Part model, mm, in its own coordinate system. A direction names the side the tool comes from. Give positions to 0.01 mm unless a question says otherwise; leave off trailing zeros. Order: outer loops, then holes, each group sorted by start corner. A loop starts at its lowest first (then second) coordinate and runs counter-clockwise, first axis right, second up. Notation, with made-up numbers: (46.5, -4) - (93.5, -4) arc R20 cw to (93.5, 25) - close; hole circle Ø6 at (81.5, -17.75). An arc over 180 degrees is marked (long way). Use one line per item in the form item = value. Start each with the question number.
1. Pin check, flat tips, straight feed: P1, Ø21, axis at x = -3, y = -9.5, coming from the +Z side; P2, Ø12, axis at y = -25, z = 8.5, coming from the -X side; P3, Ø1.5, axis at x = -2.5, z = 19, coming from the +Y side; P4, Ø5, axis at y = -9.5, z = 7.5, coming from the +X side. Stop position of each tip, or through.
2. Tool access for faces 5 (the face through (-44.365, -29.068, 1.521)), 6 (the face through (-1, 0, 3)): list every direction of +Z, -Z, +X, -X, +Y, -Y with a clear straight run to the whole face (end or side of a thin tool).
3. Band-saw the part on B-B, the plane y = -20. State how many separate pieces and enclosed holes the cut face has, plus the area to 3 significant figures.
4. Drill centre lines: line 1 (Y direction, x = -30, z = 2.2); line 2 (Z direction, x = 22.5, y = 14); line 3 (X direction, y = -6.5, z = 11). Where is each one in solid material? Low to high.
5. Band-saw the part on A-A, the plane z = 14.25. List the corners of the cut face in (x, y).
6. Pull direction Y, two halves, no side cores. Call faces 1 (the face through (31.88, -1.37, 22.84)), 2 (the face through (-28.092, -19.399, 1.521)), 3 (the face through (31.908, -19.399, 1.521)), 4 (the face through (-44.14, 34.1, 1.52)): +Y half, -Y half, draft (parallel to the pull), parting line (faces both ways), or undercut.
from build123d import *

# Parameters (mm, degrees)
SKETCH_2_W          = 90
SKETCH_2_H          = 70
EXTRUDE_2_DEPTH     = 3
SKETCH_3_R          = 2
CUT_EXTRUDE_1_DEPTH = 3
SKETCH_4_R          = 32.75
SKETCH_4_R_2        = 30.75
EXTRUDE_3_DEPTH     = 20
SKETCH_5_W          = 3
SKETCH_5_H          = 4
CUT_EXTRUDE_2_DEPTH = 20
CHAMFER_1_SIZE      = 1
CHAMFER_2_SIZE      = 1
CHAMFER_2_SIZE_2    = 1.07199294
FILLET_1_R          = 3
CUT_EXTRUDE_START   = -4
CUT_EXTRUDE_3_DEPTH = 5
FILLET_2_R          = 3


with BuildPart() as part:
    # 草图2 → 凸台-拉伸2 (new body)
    with BuildSketch(Plane.XY):
        Rectangle(SKETCH_2_W, SKETCH_2_H)
    extrude(amount=EXTRUDE_2_DEPTH)

    # 草图3 → 切除-拉伸1 (cut)
    with BuildSketch(Plane.XY.offset(3)):
        with Locations((-30, 20)):
            Circle(SKETCH_3_R)
        with Locations((-30, -20)):
            Circle(SKETCH_3_R)
        with Locations((30, -20)):
            Circle(SKETCH_3_R)
        with Locations((30, 20)):
            Circle(SKETCH_3_R)
    extrude(amount=-CUT_EXTRUDE_1_DEPTH, mode=Mode.SUBTRACT)

    # 草图4 → 凸台-拉伸3 (add)
    with BuildSketch(Plane.XY.offset(3)):
        Circle(SKETCH_4_R)
        Circle(SKETCH_4_R_2, mode=Mode.SUBTRACT)
    extrude(amount=EXTRUDE_3_DEPTH)

    # 草图5 → 切除-拉伸2 (cut)
    with BuildSketch(Plane.XY.offset(23)):
        with Locations((-31.5, 0)):
            Rectangle(SKETCH_5_W, SKETCH_5_H)
    extrude(amount=-CUT_EXTRUDE_2_DEPTH, mode=Mode.SUBTRACT)

    # 倒角1
    chamfer_1_edges = [part.edges().sort_by_distance(p)[0] for p in [
        (1.000466936, -32.734714997, 23),
        (1.000529767, 30.733718294, 23),
    ]]
    chamfer(chamfer_1_edges, length=CHAMFER_1_SIZE - 0.0001)  # a hair under: the kernel refuses the full size

    # 倒角2
    # the kernel refuses this chamfer: 1.07199294, 1, 0.94410674 mm, written as the material it takes off along each edge
    with BuildSketch(Plane(origin=(-32.688874254, -2, 24.571782988), x_dir=(0.07527193503406021, -0.997163043737697, 0), z_dir=(0, 0, -1))) as chamfer_2_piece_1:
        with BuildLine():
            Line((0.932457463, 0), (CHAMFER_2_SIZE * 0.0752719350341, -CHAMFER_2_SIZE * 0.997163043738))
            Line((CHAMFER_2_SIZE * 0.0752719350341, -CHAMFER_2_SIZE * 0.997163043738), (0, 0))
            ThreePointArc((0, 0), (0.479261525, 0.003316189), (0.932457463, 0))
        make_face()
    extrude(amount=21.571782988, mode=Mode.SUBTRACT)
    with BuildSketch(Plane(origin=(-30.684890419, -2, 24.761558832), x_dir=(-1, 0, 0), z_dir=(0, 0, -1))) as chamfer_2_piece_2:
        with BuildLine():
            Line((CHAMFER_2_SIZE_2, 0), (-0.08291501, -1.013569498))
            ThreePointArc((-0.08291501, -1.013569498), (-0.038528119, -0.522494358), (0, 0))
            Line((0, 0), (CHAMFER_2_SIZE_2, 0))
        make_face()
    extrude(amount=21.761558832, mode=Mode.SUBTRACT)
    with BuildSketch(Plane(origin=(-32.688874254, 2, 24.571782988), x_dir=(1, 0, 0), z_dir=(0, 0, -1))) as chamfer_2_piece_3:
        with BuildLine():
            Line((CHAMFER_2_SIZE, 0), (0.070187878, -0.929812122))
            ThreePointArc((0.070187878, -0.929812122), (0.032768161, -0.478151497), (0, 0))
            Line((0, 0), (CHAMFER_2_SIZE, 0))
        make_face()
    extrude(amount=21.571782988, mode=Mode.SUBTRACT)
    with BuildSketch(Plane(origin=(-30.684890419, 2, 24.761558832), x_dir=(0.08153260293948016, 0.9966706751269013, 0), z_dir=(0, 0, -1))) as chamfer_2_piece_4:
        with BuildLine():
            Line((1.016955273, 0), (-CHAMFER_2_SIZE_2 * 0.081532602904, -CHAMFER_2_SIZE_2 * 0.996670674693))
            Line((-CHAMFER_2_SIZE_2 * 0.081532602904, -CHAMFER_2_SIZE_2 * 0.996670674693), (0, 0))
            ThreePointArc((0, 0), (0.523896102, -0.004200479), (1.016955273, 0))
        make_face()
    extrude(amount=21.761558832, mode=Mode.SUBTRACT)

    # 圆角1
    fillet_1_edges = [part.edges().sort_by_distance(p)[0] for p in [
        (-45, 35, 1.5),
        (45, 35, 1.5),
        (45, -35, 1.5),
        (-45, -35, 1.5),
    ]]
    fillet(fillet_1_edges, radius=FILLET_1_R)

    # 切除-拉伸3: read off the stored shape, not the designer's step
    # 切除-拉伸3 outline → 切除-拉伸3 (cut)
    with BuildSketch(Plane.XY.offset(3).offset(CUT_EXTRUDE_START)):
        with BuildLine():
            Line((45, -32), (45, -29.59414942))
            ThreePointArc((45, -29.59414942), (22.661769286, -33.643696457), (-7.97e-07, -35))
            Line((-7.97e-07, -35), (42, -35))
            ThreePointArc((42, -35), (44.121320344, -34.121320344), (45, -32))
        make_face()
        with BuildLine():
            Line((-42, -35), (-7.97e-07, -35))
            ThreePointArc((-7.97e-07, -35), (-22.661770078, -33.643696362), (-45, -29.59414942))
            Line((-45, -29.59414942), (-45, -32))
            ThreePointArc((-45, -32), (-44.121320344, -34.121320344), (-42, -35))
        make_face()
    extrude(amount=CUT_EXTRUDE_3_DEPTH, mode=Mode.SUBTRACT)

    # 圆角2
    fillet_2_edges = [part.edges().sort_by_distance(p)[0] for p in [
        (45, -29.59414942, 1.5),
        (-45, -29.59414942, 1.5),
    ]]
    fillet(fillet_2_edges, radius=FILLET_2_R)


solid = part.part
From the geometry:
q1.P1 = 3
q1.P2 = -45
q1.P3 = 32.7
q1.P4 = 31.99
q2.face_5 = +Z, -Z, -X, -Y
q2.face_6 = +Z
q3.separate_pieces = 3
q3.enclosed_holes = 0
q3.area = 346 mm²
q4.line_1 = -32.62 to -22, -18 to 18, 22 to 35
q4.line_2 = 0 to 3
q4.line_3 = -32.1 to -30.06, 30.06 to 32.1
q5.outline = (-32.62, -2.93) arc R32.75 ccw (long way) to (-32.62, 2.93) - (-31.72, 2.03) - (-30.6, 3.01) arc R30.75 cw (long way) to (-30.6, -3.01) - (-31.72, -2.03) - close
q6.face_1 = parting line
q6.face_2 = undercut
q6.face_3 = undercut
q6.face_4 = +Y half
